Design review of the part shown in the three views and the two pictorial views. Dimensions are in mm from the part's minimum x, y and z. Give positions to 0.01 mm unless a question says otherwise; leave off trailing zeros. Loops run counter-clockwise (first coordinate to the right, second up) from the corner with the lowest first, then second, coordinate; pieces in that order, holes last. Notation, with made-up numbers: (-2, 74.25) - (35, 74.25) arc R26 ccw to (35, 100.25) - close; hole circle Ø4 at (-7, 37). An arc over 180 degrees is marked (long way). Answer as a JSON object with one key per item and string values.
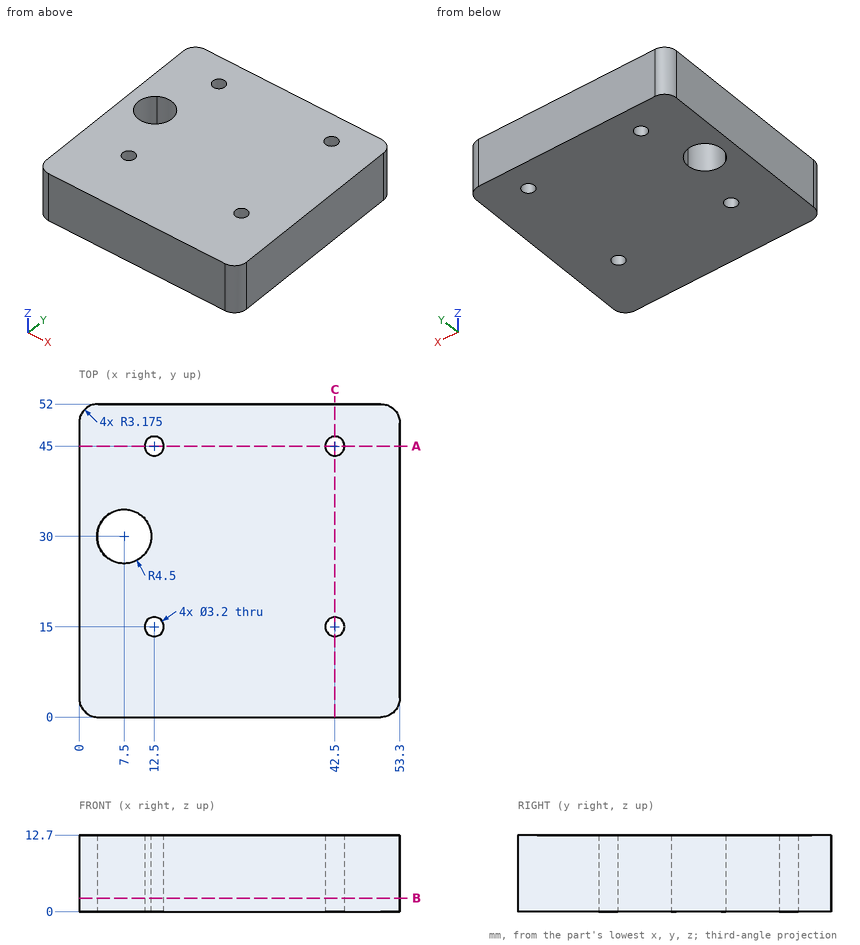
Q1. Consider section A-A, the plane y = 45. State the section outline as (x, z) points.
Results:
{"outline": "(0, 0) - (10.9, 0) - (10.9, 12.7) - (0, 12.7) - close; (14.1, 0) - (40.9, 0) - (40.9, 12.7) - (14.1, 12.7) - close; (44.1, 0) - (53.3, 0) - (53.3, 12.7) - (44.1, 12.7) - close"}
Q2. Consider section B-B, the plane z = 2.25. State the section outline as (x, y) points (3 decimals).
Results:
{"outline": "(0, 3.175) arc R3.175 ccw to (3.175, 0) - (50.125, 0) arc R3.175 ccw to (53.3, 3.175) - (53.3, 48.825) arc R3.175 ccw to (50.125, 52) - (3.175, 52) arc R3.175 ccw to (0, 48.825) - close; hole circle Ø9 at (7.5, 30); hole circle Ø3.2 at (12.5, 15); hole circle Ø3.2 at (12.5, 45); hole circle Ø3.2 at (42.5, 15); hole circle Ø3.2 at (42.5, 45)"}
Q3. To check wall thickness, follow probe 1 along Y at (x, z) = (12.5, 10); probe 2 along Y at (x, z) = (10, 1.5); probe 3 along Y at (x, z) = (11.5, 9.75). State the ranges of each line that lie inside material, in increasing order. Write a range as [from, to].
Results:
{"probe 1": "y = [0, 13.4], [16.6, 43.4], [46.6, 52]", "probe 2": "y = [0, 26.26], [33.74, 52]", "probe 3": "y = [0, 13.75], [16.25, 27.94], [32.06, 43.75], [46.25, 52]"}
Q4. Consider section C-C, the plane x = 42.5. State the section outline as (y, z) points, plus the area to 3 significant figures.
Results:
{"outline": "(0, 0) - (13.4, 0) - (13.4, 12.7) - (0, 12.7) - close; (16.6, 0) - (43.4, 0) - (43.4, 12.7) - (16.6, 12.7) - close; (46.6, 0) - (52, 0) - (52, 12.7) - (46.6, 12.7) - close", "area": "579 mm^2"}
